Autodesk Inventor part; units mm, degrees
ref_plane "YZ Plane" through (0, 0, 0) normal (1, 0, 0) x (0, 1, 0)
ref_plane "XZ Plane" through (0, 0, 0) normal (0, 1, 0) x (-1, 0, 0)
ref_plane "XY Plane" through (0, 0, 0) normal (0, 0, 1) x (1, 0, 0)
sketch "Sketch1" plane through (0, 0, 0) normal (0, 0, 1) x (1, 0, 0)
  line L0 (0, 0) -> (6, 0)
  line L1 (6, 0) -> (6, 11)
  line L2 (0, 0) -> (-6, 0)
  line L3 (-6, 0) -> (-6, 11)
  line L4 (0, 0) -> (0, 15)
  line L5 (0, 15) -> (2, 15)
  line L6 (2, 15) -> (6, 11)
  line L7 (0, 15) -> (-2, 15)
  line L8 (-2, 15) -> (-6, 11)
  dimension "d0" = 6
  dimension "d1" = 11
  dimension "d2" = 6
  dimension "d3" = 11
  dimension "d4" = 15
  dimension "d5" = 2
  dimension "d6" = 2
extrude "Extrusion1" add sketch "Sketch1" along normal blind 6
sketch "Sketch2" plane through (6, 0, 0) normal (1, 0, 0) x (0, 0, -1)
  line L0 (0, 11) -> (0, 15)
  line L1 (0, 0) -> (0, 15)
  line L2 (0, 15) -> (-2, 15)
  line L3 (0, 15) -> (-6, 15)
  line L4 (0, 11) -> (0, 0)
  line L5 (0, 0) -> (-0.4, 0)
  line L6 (0, 0) -> (-6, 0)
  line L7 (-2, 15) -> (-2.4, 15)
  line L8 (-2.4, 15) -> (-0.4, 0)
  dimension "d9" = 2
extrude "Extrusion2" cut sketch "Sketch2" against normal blind 17.9375
properties part number "middle-join-inside"
Read the model definition and answer for the solid it produces. Units are mm, in the model's axes. Round coordinates to 2 decimals unless told otherwise and drop trailing zeros. Write each loop counter-clockwise with the first axis right and the second up, starting at its lowest first coordinate (ties: lowest second). Pieces come first, ordered by that corner, then holes.
1. Given pin 1 Ø1.5 at (x, y) = (0, 8) entering from -Z, flat-ended and moving along its own axis, determine where the tip first touches the part or whether it passes through.
2. The part is cut by section A-A, the plane x = 1.25. Determine the outline of the cut face in (y, z).
3. Determine the mould class of faces 1 (the face through (0, 8, 6)), 2 (the face through (6, 5, 4)), 3 (the face through (-6, 5, 4)) for opening direction X: pulls with the +X half, pulls with the -X half, needs draft (parallel to the pull), parting line crosses it, or undercut.
4. Straight lines are drawn through the part: L1, parallel to X at y = 13.5, z = 5.75; L2, parallel to Z at x = 1.25, y = 10; L3, parallel to Z at x = -5.5, y = 4.75. For each, find the intervals that lie inside material, in ascending order.
5. The part is cut by section C-C, the plane z = 3.05. Determine the outline of the cut face in (x, y).
6. The part is cut by section B-B, the plane z = 1.6. Determine the outline of the cut face in (x, y).
Values:
1. pin 1: stops at z = 1.37
2. outline: (0, 0.4) - (15, 2.4) - (15, 6) - (0, 6) - close
3. face 1: needs draft
3. face 2: pulls with the +X half
3. face 3: pulls with the -X half
4. L1: x = -3.5 to 3.5
4. L2: z = 1.73 to 6
4. L3: z = 1.03 to 6
5. outline: (-6, 0) - (6, 0) - (6, 11) - (2, 15) - (-2, 15) - (-6, 11) - close
6. outline: (-6, 0) - (6, 0) - (6, 9) - (-6, 9) - close
